For this review, use the dimensioned drawing (mm, ordinates from the lowest corner) and the shaded views. Round coordinates to 2 decimals unless told otherwise and drop trailing zeros. Order: outer loops, then holes, each group sorted by start corner. A loop starts at its lowest first (then second) coordinate and runs counter-clockwise, first axis right, second up. Notation, with made-up numbers: (73, 71) -> (98, 71) arc R28 ccw to (98, 97) -> close; hole circle Ø4 at (11.25, 46). An arc over 180 degrees is marked (long way). Use a Markdown table: item, result. Add a question column.
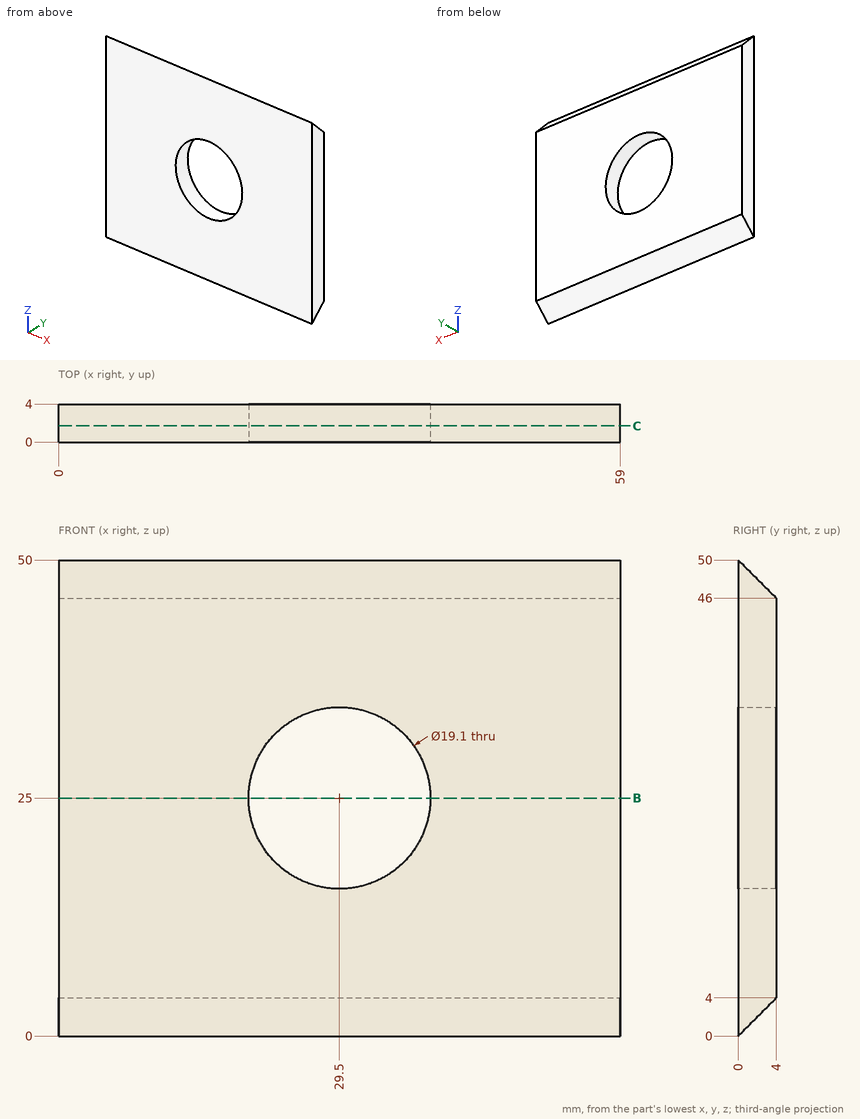
Q1. Wall thickness on line 1 (X direction, y = 1.55, z = 25); line 2 (X direction, y = 2.85, z = 30); line 3 (Z direction, x = 31.5, y = 3.2): over which ranges is each line inside the solid? List them lowest first. Write a range as [from, to].
Q2. Insertion check: pin 1 (1.5 mm diameter, centred on x = 23.5, y = 2, fed in from -Z). The pin has a flat end and moves straight along its axis. Give the tip position at first contact, or say it passes through.
Q3. Add section B-B (z = 25). Write out the cut boundary in (x, y), then the cut area to 3 significant figures.
Q4. Add section C-C (y = 1.7). Write out the cut boundary in (x, z), then the cut area to 3 significant figures.
Report:
| question | item | result |
|---|---|---|
| 1 | line 1 | x = [0, 19.95], [39.05, 59] |
| 1 | line 2 | x = [0, 21.36], [37.64, 59] |
| 1 | line 3 | z = [3.2, 15.66], [34.34, 46.8] |
| 2 | pin 1 | stops at z = 1.25 |
| 3 | outline | (0, 0) -> (19.95, 0) -> (19.95, 4) -> (0, 4) -> close; (39.05, 0) -> (59, 0) -> (59, 4) -> (39.05, 4) -> close |
| 3 | area | 160 mm² |
| 4 | outline | (0, 1.7) -> (59, 1.7) -> (59, 48.3) -> (0, 48.3) -> close; hole circle Ø19.1 at (29.5, 25) |
| 4 | area | 2,460 mm² |
